from build123d import *

# Parameters (mm, degrees)
SKETCH1_R                 = 38.1
BOSS_EXTRUDE1_DEPTH       = 6.35
F_1_4_20_TAPPED_HOLE1_D   = 5.1054
F_8_CLEARANCE_HOLE1_D     = 4.4958
F_8_CLEARANCE_HOLE1_DEPTH = 313.436
F_8_CLEARANCE_HOLE1_TIP   = 1.350674586


with BuildPart() as part:
    # Sketch1 → Boss-Extrude1 (new body)
    with BuildSketch(Plane.XY):
        Circle(SKETCH1_R)
    extrude(amount=BOSS_EXTRUDE1_DEPTH)

    # 1/4-20 Tapped Hole1 (through all)
    with Locations(Plane.XY.offset(6.35)):
        with Locations((0, 0)):
            Hole(F_1_4_20_TAPPED_HOLE1_D / 2)

    # #8 Clearance Hole1
    with Locations(Plane.XY.offset(6.35)):
        with Locations((-31.75, 0), (-27.49630657, 15.875), (-15.875, 27.49630657), (0, 31.75), (15.875, 27.49630657), (27.49630657, 15.875), (31.75, 0), (27.49630657, -15.875), (15.875, -27.49630657), (0, -31.75), (-15.875, -27.49630657), (-27.49630657, -15.875)):
            Hole(F_8_CLEARANCE_HOLE1_D / 2, depth=F_8_CLEARANCE_HOLE1_DEPTH)
            with Locations((0, 0, -(F_8_CLEARANCE_HOLE1_DEPTH + F_8_CLEARANCE_HOLE1_TIP / 2))):  # 118° drill point
                Cone(0, F_8_CLEARANCE_HOLE1_D / 2, F_8_CLEARANCE_HOLE1_TIP, mode=Mode.SUBTRACT)


solid = part.part
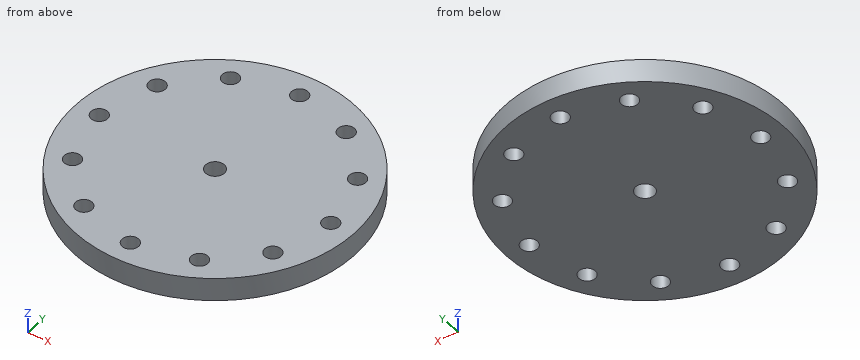
Build history of the part. All positions in model axes, mm. Round coordinates to 2 decimals unless told otherwise and drop trailing zeros. Loops run counter-clockwise (first coordinate to the right, second up) from the corner with the lowest first, then second, coordinate; pieces in that order, holes last. Notation, with made-up numbers: (89.5, 84) -> (128.5, 84) arc R28 cw to (128.5, 120) -> close; hole circle Ø4 at (37, 48). An arc over 180 degrees is marked (long way). Use CSV: the item, a comma, the result in double quotes. Start each with the question number.
Q1. Saw through at C-C on z = 3.5. Count the separate pieces of the cut face and the enclosed holes in it, and give its area (3 significant figures).
Q2. Flat gauge pins, fed straight in: pin 1 Ø2 at (y, z) = (24, 4) entering from -X; pin 2 Ø1.5 at (y, z) = (-25.5, 2) entering from -X; pin 3 Ø1 at (x, z) = (18.5, 3) entering from +Y. Where does each tip first touch, or does it go through?
Q3. Saw through at A-A on y = 0. Give the cut face in (x, z).
Q4. Saw through at B-B on x = 31.75. Give the cut face in (y, z).
Q5. Drill centre lines: L1, parallel to Y at x = 0, z = 2; L2, parallel to X at y = 1.5, z = 1; L3, parallel to Y at x = 14, z = 4.25. Where is each one in solid material? Low to high.
Solutions:
1,separate pieces,"1"
1,enclosed holes,"13"
1,area,"4,350 mm^2"
2,pin 1,"stops at x = -30.37"
2,pin 2,"stops at x = -28.97"
2,pin 3,"stops at y = 33.58"
3,outline,"(-38.1, 0) -> (-34, 0) -> (-34, 6.35) -> (-38.1, 6.35) -> close; (-29.5, 0) -> (-2.55, 0) -> (-2.55, 6.35) -> (-29.5, 6.35) -> close; (2.55, 0) -> (29.5, 0) -> (29.5, 6.35) -> (2.55, 6.35) -> close; (34, 0) -> (38.1, 0) -> (38.1, 6.35) -> (34, 6.35) -> close"
4,outline,"(-21.06, 0) -> (-2.25, 0) -> (-2.25, 6.35) -> (-21.06, 6.35) -> close; (2.25, 0) -> (21.06, 0) -> (21.06, 6.35) -> (2.25, 6.35) -> close"
5,L1,"y = -38.1 to -34, -29.5 to -2.55, 2.55 to 29.5, 34 to 38.1"
5,L2,"x = -38.07 to -33.42, -30.08 to -2.07, 2.07 to 30.08, 33.42 to 38.07"
5,L3,"y = -35.43 to -28.74, -26.26 to 26.26, 28.74 to 35.43"
